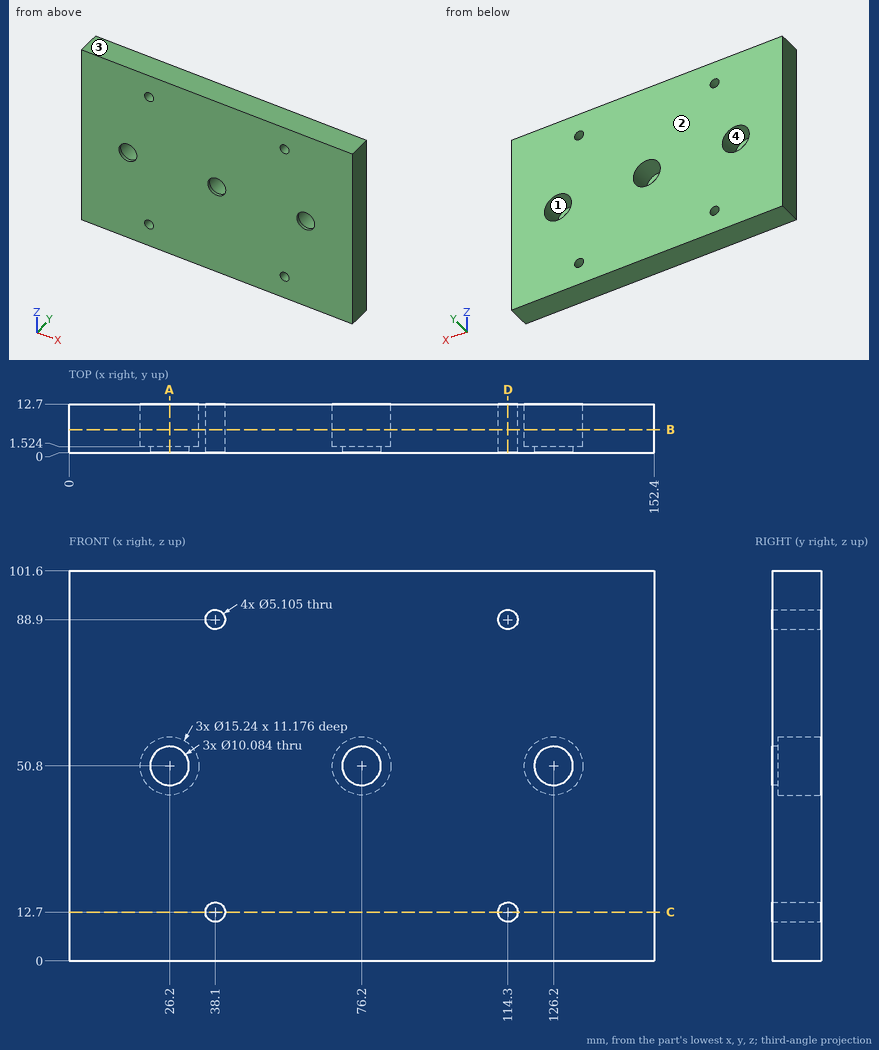
The figure shows three views and two pictorial views of one solid part (mm, origin at its lowest corner). Answer the questions. A direction names the side the tool comes from. Coordinates: 2 decimals unless noted, no trailing zeros. Write each loop counter-clockwise with the first axis right and the second up, starting at its lowest first coordinate (ties: lowest second). Pieces come first, ordered by that corner, then holes. Notation, with made-up numbers: (43, -10) -> (49, -10) arc R18 ccw to (49, 5) -> close; hole circle Ø9 at (29, -26.5). An arc over 180 degrees is marked (long way). Answer as a JSON object with one key per item and string values.
Q1. Consider line 1 (Z direction, x = 38.1, y = 7.5); line 2 (Z direction, x = 76.2, y = 0.55); line 3 (X direction, y = 9.25, z = 54.5). Determine where each line is inside the solid, lowest interval first. Write a range as [from, to].
The answers:
{"line 1": "z = [0, 10.15], [15.25, 86.35], [91.45, 101.6]", "line 2": "z = [0, 45.76], [55.84, 101.6]", "line 3": "x = [0, 19.54], [32.86, 69.54], [82.86, 119.54], [132.86, 152.4]"}
Q2. Determine the mould class of the marked faces 3 and 4 for opening direction X: pulls with the +X half, pulls with the -X half, needs draft (parallel to the pull), parting line crosses it, or undercut.
The answers:
{"face 3": "needs draft", "face 4": "undercut"}
Q3. A tool of negligible diameter and unlimited length cuts with its end or side. For the marked faces 1 and 2, from which of +Z, -Z, +X, -X, +Y, -Y can it reach the whole face along a straight path? Write none if from no direction.
The answers:
{"face 1": "+Y", "face 2": "+Z, -Z, +X, -X, +Y"}
Q4. The part is cut by section B-B on y = 6. Give the vertices of the cut face in (x, z) (1 decimal).
The answers:
{"outline": "(0, 0) -> (152.4, 0) -> (152.4, 101.6) -> (0, 101.6) -> close; hole circle Ø15.2 at (26.2, 50.8); hole circle Ø5.1 at (38.1, 12.7); hole circle Ø5.1 at (38.1, 88.9); hole circle Ø15.2 at (76.2, 50.8); hole circle Ø5.1 at (114.3, 12.7); hole circle Ø5.1 at (114.3, 88.9); hole circle Ø15.2 at (126.2, 50.8)"}
Q5. A flat-ended cylindrical pin translates along its axis: pin 1 Ø7.5 at (x, z) = (75, 48.5) entering from +Y. Find the tip coordinate at first contact, or state that the pin passes through.
The answers:
{"pin 1": "stops at y = 1.52"}
Q6. The part is cut by section D-D on x = 114.3. Give the vertices of the cut face in (y, z).
The answers:
{"outline": "(0, 0) -> (12.7, 0) -> (12.7, 10.15) -> (0, 10.15) -> close; (0, 15.25) -> (12.7, 15.25) -> (12.7, 86.35) -> (0, 86.35) -> close; (0, 91.45) -> (12.7, 91.45) -> (12.7, 101.6) -> (0, 101.6) -> close"}
Q7. The part is cut by section A-A on x = 26.2. Give the vertices of the cut face in (y, z), then the cut area to 3 significant figures.
The answers:
{"outline": "(0, 0) -> (12.7, 0) -> (12.7, 43.18) -> (1.52, 43.18) -> (1.52, 45.76) -> (0, 45.76) -> close; (0, 55.84) -> (1.52, 55.84) -> (1.52, 58.42) -> (12.7, 58.42) -> (12.7, 101.6) -> (0, 101.6) -> close", "area": "1,100 mm2"}
Q8. The part is cut by section C-C on z = 12.7. Give the vertices of the cut face in (x, y), then the cut area to 3 significant figures.
The answers:
{"outline": "(0, 0) -> (35.55, 0) -> (35.55, 12.7) -> (0, 12.7) -> close; (40.65, 0) -> (111.75, 0) -> (111.75, 12.7) -> (40.65, 12.7) -> close; (116.85, 0) -> (152.4, 0) -> (152.4, 12.7) -> (116.85, 12.7) -> close", "area": "1,810 mm2"}
